```python
from build123d import *

# Parameters (mm, degrees)
F1_DEPTH = 70
F2_R     = 1.25
F2_W     = 20.9
F2_H     = 3.6
F3_DEPTH = 4
F4_DEPTH = 1
F2_W_2   = 2
F2_H_2   = 1.2
F5_DEPTH = 1.5


with BuildPart() as f1:
    # F0 (on Right) → F1 (new body, symmetric)
    with BuildSketch(Plane.YZ):
        Polygon((-1.6, 10.55), (-1.6, 0), (-1.6, -10.55), (-0.7, -10.55), (-0.7, -12.55), (-1.6, -12.55), (-1.6, -13.55), (0, -13.55), (1.6, -13.55), (1.6, -12.55), (0.7, -12.55), (0.7, -10.55), (1.6, -10.55), (1.6, 0), (1.6, 10.55), (0.7, 10.55), (0.7, 12.55), (1.6, 12.55), (1.6, 13.55), (0, 13.55), (-1.6, 13.55), (-1.6, 12.55), (-0.7, 12.55), (-0.7, 10.55), align=None)
    extrude(amount=F1_DEPTH, both=True)

    # F2 (on face) → F3 (cut)
    with BuildSketch(Plane.XZ.offset(1.6)):
        with BuildLine():
            Line((-7, -4.05), (-4, -4.05))
            ThreePointArc((-4, -4.05), (-3.646447, -3.903553), (-3.5, -3.55))
            Line((-3.5, -3.55), (-3.5, -0.55))
            ThreePointArc((-3.5, -0.55), (-3.646447, -0.196447), (-4, -0.05))
            Line((-4, -0.05), (-7, -0.05))
            ThreePointArc((-7, -0.05), (-7.353553, -0.196447), (-7.5, -0.55))
            Line((-7.5, -0.55), (-7.5, -3.55))
            ThreePointArc((-7.5, -3.55), (-7.353553, -3.903553), (-7, -4.05))
        make_face()
        with BuildLine():
            ThreePointArc((1.5, -0.55), (1.353553, -0.196447), (1, -0.05))
            Line((1, -0.05), (-2, -0.05))
            ThreePointArc((-2, -0.05), (-2.353553, -0.196447), (-2.5, -0.55))
            Line((-2.5, -0.55), (-2.5, -3.55))
            ThreePointArc((-2.5, -3.55), (-2.353553, -3.903553), (-2, -4.05))
            Line((-2, -4.05), (1, -4.05))
            ThreePointArc((1, -4.05), (1.353553, -3.903553), (1.5, -3.55))
            Line((1.5, -3.55), (1.5, -0.55))
        make_face()
        with BuildLine():
            ThreePointArc((6.5, -0.55), (6.353553, -0.196447), (6, -0.05))
            Line((6, -0.05), (3, -0.05))
            ThreePointArc((3, -0.05), (2.646447, -0.196447), (2.5, -0.55))
            Line((2.5, -0.55), (2.5, -3.55))
            ThreePointArc((2.5, -3.55), (2.646447, -3.903553), (3, -4.05))
            Line((3, -4.05), (6, -4.05))
            ThreePointArc((6, -4.05), (6.353553, -3.903553), (6.5, -3.55))
            Line((6.5, -3.55), (6.5, -0.55))
        make_face()
        with BuildLine():
            ThreePointArc((11.5, -0.55), (11.353553, -0.196447), (11, -0.05))
            Line((11, -0.05), (8, -0.05))
            ThreePointArc((8, -0.05), (7.646447, -0.196447), (7.5, -0.55))
            Line((7.5, -0.55), (7.5, -3.55))
            ThreePointArc((7.5, -3.55), (7.646447, -3.903553), (8, -4.05))
            Line((8, -4.05), (11, -4.05))
            ThreePointArc((11, -4.05), (11.353553, -3.903553), (11.5, -3.55))
            Line((11.5, -3.55), (11.5, -0.55))
        make_face()
        with BuildLine():
            ThreePointArc((16.5, -0.55), (16.353553, -0.196447), (16, -0.05))
            Line((16, -0.05), (13, -0.05))
            ThreePointArc((13, -0.05), (12.646447, -0.196447), (12.5, -0.55))
            Line((12.5, -0.55), (12.5, -3.55))
            ThreePointArc((12.5, -3.55), (12.646447, -3.903553), (13, -4.05))
            Line((13, -4.05), (16, -4.05))
            ThreePointArc((16, -4.05), (16.353553, -3.903553), (16.5, -3.55))
            Line((16.5, -3.55), (16.5, -0.55))
        make_face()
        with BuildLine():
            ThreePointArc((21.5, -0.55), (21.353553, -0.196447), (21, -0.05))
            Line((21, -0.05), (18, -0.05))
            ThreePointArc((18, -0.05), (17.646447, -0.196447), (17.5, -0.55))
            Line((17.5, -0.55), (17.5, -3.55))
            ThreePointArc((17.5, -3.55), (17.646447, -3.903553), (18, -4.05))
            Line((18, -4.05), (21, -4.05))
            ThreePointArc((21, -4.05), (21.353553, -3.903553), (21.5, -3.55))
            Line((21.5, -3.55), (21.5, -0.55))
        make_face()
        with BuildLine():
            ThreePointArc((26.5, -0.55), (26.353553, -0.196447), (26, -0.05))
            Line((26, -0.05), (23, -0.05))
            ThreePointArc((23, -0.05), (22.646447, -0.196447), (22.5, -0.55))
            Line((22.5, -0.55), (22.5, -3.55))
            ThreePointArc((22.5, -3.55), (22.646447, -3.903553), (23, -4.05))
            Line((23, -4.05), (26, -4.05))
            ThreePointArc((26, -4.05), (26.353553, -3.903553), (26.5, -3.55))
            Line((26.5, -3.55), (26.5, -0.55))
        make_face()
        with BuildLine():
            Line((32.9, -4.05), (39.1, -4.05))
            ThreePointArc((39.1, -4.05), (39.807107, -3.757107), (40.1, -3.05))
            Line((40.1, -3.05), (40.1, -0.85))
            ThreePointArc((40.1, -0.85), (39.807107, -0.142893), (39.1, 0.15))
            Line((39.1, 0.15), (32.9, 0.15))
            ThreePointArc((32.9, 0.15), (32.192893, -0.142893), (31.9, -0.85))
            Line((31.9, -0.85), (31.9, -3.05))
            ThreePointArc((31.9, -3.05), (32.192893, -3.757107), (32.9, -4.05))
        make_face()
        with BuildLine():
            Line((47.8, -4.05), (58.6, -4.05))
            ThreePointArc((58.6, -4.05), (60.014214, -3.464214), (60.6, -2.05))
            Line((60.6, -2.05), (60.6, 1.45))
            ThreePointArc((60.6, 1.45), (60.014214, 2.864214), (58.6, 3.45))
            Line((58.6, 3.45), (47.8, 3.45))
            ThreePointArc((47.8, 3.45), (46.385786, 2.864214), (45.8, 1.45))
            Line((45.8, 1.45), (45.8, -2.05))
            ThreePointArc((45.8, -2.05), (46.385786, -3.464214), (47.8, -4.05))
        make_face()
        with Locations((-33.9, -7.9)):
            Circle(F2_R)
        with Locations((-20.65, -8.15)):
            Rectangle(F2_W, F2_H)
        with Locations((-47.65, -8.15)):
            Rectangle(F2_W, F2_H)
        with Locations((-60.9, -7.9)):
            Circle(F2_R)
    extrude(amount=-F3_DEPTH, mode=Mode.SUBTRACT)

    # F2 (on face) → F4 (cut)
    with BuildSketch(Plane.XZ.offset(1.6)):
        Polygon((-10.2, -9.95), (-9.2, -9.95), (-9.2, -5.85), (-63, -5.85), (-63, -9.95), (-58.1, -9.95), (-58.1, -6.35), (-37.2, -6.35), (-37.2, -9.95), (-31.1, -9.95), (-31.1, -6.35), (-10.2, -6.35), align=None)
        with Locations((-60.9, -7.9)):
            Circle(F2_R, mode=Mode.SUBTRACT)
        with Locations((-33.9, -7.9)):
            Circle(F2_R, mode=Mode.SUBTRACT)
    extrude(amount=-F4_DEPTH, mode=Mode.SUBTRACT)

    # F2 (on face) → F5 (join)
    with BuildSketch(Plane.XZ.offset(1.6)):
        with Locations((-66.8, -3.35)):
            Rectangle(F2_W_2, F2_H_2)
        with Locations((-66.8, -6.55)):
            Rectangle(F2_W_2, F2_H_2)
        with Locations((-34, -3.35)):
            Rectangle(F2_W_2, F2_H_2)
        with Locations((-11, -3.35)):
            Rectangle(F2_W_2, F2_H_2)
        with Locations((-4, -6.55)):
            Rectangle(F2_W_2, F2_H_2)
        with Locations((25, -6.55)):
            Rectangle(F2_W_2, F2_H_2)
        with Locations((29.5, -3.35)):
            Rectangle(F2_W_2, F2_H_2)
        with Locations((43.3, -3.35)):
            Rectangle(F2_W_2, F2_H_2)
        with Locations((48.5, -6.55)):
            Rectangle(F2_W_2, F2_H_2)
        with Locations((65.5, -3.35)):
            Rectangle(F2_W_2, F2_H_2)
        with Locations((65.5, -6.55)):
            Rectangle(F2_W_2, F2_H_2)
    extrude(amount=F5_DEPTH)


solid = f1.part
```
Source: CAD feature listing. Evaluate the final solid. Frame: model axes, mm. Round coordinates to 2 decimals unless told otherwise and drop trailing zeros. Write each loop counter-clockwise with the first axis right and the second up, starting at its lowest first coordinate (ties: lowest second). Pieces come first, ordered by that corner, then holes. Notation, with made-up numbers: M -2.75,80 L 11.25,80 A24 cw 11.25,100 Z; hole C 65,-9 d7. An arc over 180 degrees is marked long. Answer as a JSON object with one key per item and string values. Group by question number.
(1) First-contact query: pin 1 (0.6 mm diameter, centred on y = -2.5, z = -3, fed in from -X); pin 2 (10 mm diameter, centred on x = -51, z = -9.5, fed in from -Y); pin 3 (1.6 mm diameter, centred on x = 25.5, y = -2.5, fed in from +Z). Flat tips, straight axial feed; report the tip coordinate or a pass-through.
(2) Section query A-A on x = -60.9. Output: boundary loops of the cut face in (y, z), then the cut area to 3 significant figures.
(3) Section query B-B on x = -26. Output: boundary loops of the cut face in (y, z), then the cut area to 3 significant figures.
(4) Mould query, pull axis X, two halves, no side actions, for faces 1 (the flat face through (-70, 0, 0)), 2 (the flat face through (11.5, 0, -2)). Classes: +X half, -X half, draft (parallel to the pull), parting line (faces both ways), or undercut.
(5) Ray query, line 1 (Z direction, x = -15, y = 0.9); line 2 (Z direction, x = -60.9, y = 1.15); line 3 (X direction, y = -2.25, z = -3.25). Return the intervals inside material, ascending. Write a range as [from, to].
(6) Section query C-C on z = 9. Output: boundary loops of the cut face in (x, y).
Computed values:
{
 "1": {"pin 1": "x = -67.8", "pin 2": "y = -1.6", "pin 3": "z = -5.95"},
 "2": {"outline": "M -1.6,-13.55 L 1.6,-13.55 L 1.6,-12.55 L 0.7,-12.55 L 0.7,-10.55 L 1.6,-10.55 L 1.6,-9.15 L -0.6,-9.15 L -0.6,-9.95 L -1.6,-9.95 L -1.6,-10.55 L -0.7,-10.55 L -0.7,-12.55 L -1.6,-12.55 Z; M -1.6,-5.85 L -0.6,-5.85 L -0.6,-6.65 L 1.6,-6.65 L 1.6,10.55 L 0.7,10.55 L 0.7,12.55 L 1.6,12.55 L 1.6,13.55 L -1.6,13.55 L -1.6,12.55 L -0.7,12.55 L -0.7,10.55 L -1.6,10.55 Z", "area": "69.9 mm^2"},
 "3": {"outline": "M -1.6,-13.55 L 1.6,-13.55 L 1.6,-12.55 L 0.7,-12.55 L 0.7,-10.55 L 1.6,-10.55 L 1.6,-9.95 L -1.6,-9.95 L -1.6,-10.55 L -0.7,-10.55 L -0.7,-12.55 L -1.6,-12.55 Z; M -1.6,-5.85 L -0.6,-5.85 L -0.6,-6.35 L 1.6,-6.35 L 1.6,10.55 L 0.7,10.55 L 0.7,12.55 L 1.6,12.55 L 1.6,13.55 L -1.6,13.55 L -1.6,12.55 L -0.7,12.55 L -0.7,10.55 L -1.6,10.55 Z", "area": "67.5 mm^2"},
 "4": {"face 1": "-X half", "face 2": "undercut"},
 "5": {"line 1": "[-13.55, -12.55], [-10.55, -9.95], [-6.35, 10.55], [12.55, 13.55]", "line 2": "[-13.55, -12.55], [-10.55, -9.15], [-6.65, 10.55], [12.55, 13.55]", "line 3": "[-67.8, -65.8], [-35, -33], [-12, -10], [28.5, 30.5], [42.3, 44.3], [64.5, 66.5]"},
 "6": {"outline": "M -70,-1.6 L 70,-1.6 L 70,1.6 L -70,1.6 Z"}
}
